from build123d import *

# Parameters (mm, degrees)
SKETCH2_R           = 4.7625
SKETCH2_R_2         = 12.8
BOSS_EXTRUDE2_DEPTH = 5.334
SKETCH3_R           = 6.35
SKETCH3_R_2         = 4.7625
CUT_EXTRUDE3_DEPTH  = 2.667
SKETCH3_2_R         = 4.7625
CUT_EXTRUDE4_DEPTH  = 6.334


with BuildPart() as part:
    # Sketch2 → Boss-Extrude2 (new body)
    with BuildSketch(Plane.XY):
        Polygon((-24, -20.208676973), (24, -20.208676973), (68.038646731, 23.829969758), (68.038646731, 80.195030242), (24, 124.233676973), (-24, 124.233676973), (-68.038646731, 80.195030242), (-68.038646731, 23.829969758), align=None)
        Circle(SKETCH2_R, mode=Mode.SUBTRACT)
        with Locations((0, 69.35)):
            Circle(SKETCH2_R_2, mode=Mode.SUBTRACT)
        with Locations((0, 34.675)):
            Circle(SKETCH2_R_2, mode=Mode.SUBTRACT)
    extrude(amount=BOSS_EXTRUDE2_DEPTH)

    # Sketch3 → Cut-Extrude3 (cut)
    with BuildSketch(Plane.XY.offset(5.334)):
        Circle(SKETCH3_R)
        Circle(SKETCH3_R_2, mode=Mode.SUBTRACT)
        with Locations((52.0125, 52.0125)):
            Circle(SKETCH3_R)
        with Locations((52.0125, 52.0125)):
            Circle(SKETCH3_R_2, mode=Mode.SUBTRACT)
        with Locations((0, 104.025)):
            Circle(SKETCH3_R)
        with Locations((0, 104.025)):
            Circle(SKETCH3_R_2, mode=Mode.SUBTRACT)
        with Locations((-52.0125, 52.0125)):
            Circle(SKETCH3_R)
        with Locations((-52.0125, 52.0125)):
            Circle(SKETCH3_R_2, mode=Mode.SUBTRACT)
    extrude(amount=-CUT_EXTRUDE3_DEPTH, mode=Mode.SUBTRACT)

    # Sketch3_2 → Cut-Extrude4 (cut, through all)
    with BuildSketch(Plane.XY.offset(5.334)):
        with Locations((-52.0125, 52.0125)):
            Circle(SKETCH3_2_R)
        with Locations((0, 104.025)):
            Circle(SKETCH3_2_R)
        with Locations((52.0125, 52.0125)):
            Circle(SKETCH3_2_R)
    extrude(amount=-CUT_EXTRUDE4_DEPTH, mode=Mode.SUBTRACT)


solid = part.part
The model under review builds one solid part; all positions refer to its coordinate system, in mm. A direction names the side the tool comes from. Give positions to 0.01 mm unless a question says otherwise; leave off trailing zeros. Order: outer loops, then holes, each group sorted by start corner. A loop starts at its lowest first (then second) coordinate and runs counter-clockwise, first axis right, second up. Notation, with made-up numbers: M 43.25,59 L 71.25,59 A16 ccw 71.25,85 Z; hole C 34,-32 d2. An arc over 180 degrees is marked long. Answer in a Markdown table with one row per item. Add a question column.
1. Add section A-A on x = 0. Count the separate pieces of the cut face and the enclosed holes in it, plus the area to 3 significant figures.
2. Machinability: for faces 1 (the flat face through (46.328, 101.906, 2.63)), 2 (the cylindrical face through (-45.956, 53.92, 4.019)), which of the approach directions +Z, -Z, +X, -X, +Y, -Y give a long, thin tool a straight path to every point of the face, cutting with its end or side? Answer none if there is none.
3. Add section B-B on y = 54. State the section outline as (x, z) points, plus the area to 3 significant figures.
4. For pin 1 Ø1 at (x, z) = (-50.5, 1) entering from -Y; pin 2 Ø20.5 at (x, y) = (52.01, 52.01) entering from +Z; pin 3 Ø6.5 at (x, y) = (-1, -1) entering from +Z; pin 4 Ø6 at (x, y) = (-2, 101.5) entering from +Z, all flat-tipped, find the tip position at first contact; note any pin that passes through.
5. To check wall thickness, follow line 1 along Y through (x, z) = (0, 3.9) (3 decimals); line 2 along X through (y, z) = (69, 4.5); line 3 along X through (y, z) = (56, 4.25). State the ranges of each line that lie inside material, in increasing order.
6. Mouldability with a two-part tool opening along Y and no side actions: class faces 3 (the cylindrical face through (-1.666, 47.366, 2.63)), 4 (the flat face through (-1, 53, 0)), 5 (the flat face through (-45.711, 102.523, 2.63)) as released by +Y, released by -Y, zero draft, split by the parting line, or undercut.
7. Add section C-C on y = 0. State the section outline as (x, z) points, plus the area to 3 significant figures.
The answers:
| question | item | result |
|---|---|---|
| 1 | separate pieces | 5 |
| 1 | enclosed holes | 0 |
| 1 | area | 379 mm2 |
| 2 | face 1 | +Z, -Z, +X, +Y |
| 2 | face 2 | +Z |
| 3 | outline | M -68.04,0 L -56.34,0 L -56.34,2.67 L -58.04,2.67 L -58.04,5.33 L -68.04,5.33 Z; M -47.68,0 L 47.68,0 L 47.68,2.67 L 45.98,2.67 L 45.98,5.33 L -45.98,5.33 L -45.98,2.67 L -47.68,2.67 Z; M 56.34,0 L 68.04,0 L 68.04,5.33 L 58.04,5.33 L 58.04,2.67 L 56.34,2.67 Z |
| 3 | area | 615 mm2 |
| 4 | pin 1 | y = 5.79 |
| 4 | pin 2 | z = 5.33 |
| 4 | pin 3 | through |
| 4 | pin 4 | z = 2.67 |
| 5 | line 1 | -20.209 to -6.35, 6.35 to 21.875, 47.475 to 56.55, 82.15 to 97.675, 110.375 to 124.234 |
| 5 | line 2 | -68.04 to -12.8, 12.8 to 68.04 |
| 5 | line 3 | -68.04 to -56.95, -47.07 to 47.07, 56.95 to 68.04 |
| 6 | face 3 | undercut |
| 6 | face 4 | zero draft |
| 6 | face 5 | released by +Y |
| 7 | outline | M -44.21,0 L -4.76,0 L -4.76,2.67 L -6.35,2.67 L -6.35,5.33 L -44.21,5.33 Z; M 4.76,0 L 44.21,0 L 44.21,5.33 L 6.35,5.33 L 6.35,2.67 L 4.76,2.67 Z |
| 7 | area | 412 mm2 |
